```python
from build123d import *

# Parameters (mm, degrees)
F1_DEPTH  = 28.5
F2_R      = 0.5
F3_R      = 3
F4_DEPTH  = 7.9
F5_R      = 2.499
F5_R_2    = 1.999
F6_DEPTH  = 14.8
F7_R      = 2.75
F7_R_2    = 2.499
F7_R_3    = 1.999
F8_DEPTH  = 1
F10_DEPTH = 3.5
F11_R     = 0.15
F12_R     = 0.15


# Not quite as in the source:
# - a feature names something its author has since deleted; it is built from what else it names


with BuildPart() as f1:
    # F0 (on Front) → F1 (new body, symmetric)
    with BuildSketch(Plane.XZ):
        with BuildLine():
            Line((-0.9, 0.9), (-2.3313088598, 0.9))
            ThreePointArc((-2.3313088598, 0.9), (-2.499, 0), (-2.3313088598, -0.9))
            Line((-2.3313088598, -0.9), (-0.9, -0.9))
            Line((-0.9, -0.9), (-0.9, -2.3313088598))
            ThreePointArc((-0.9, -2.3313088598), (0, -2.499), (0.9, -2.3313088598))
            Line((0.9, -2.3313088598), (0.9, -0.9))
            Line((0.9, -0.9), (2.3313088598, -0.9))
            ThreePointArc((2.3313088598, -0.9), (2.499, 0), (2.3313088598, 0.9))
            Line((2.3313088598, 0.9), (0.9, 0.9))
            Line((0.9, 0.9), (0.9, 2.3313088598))
            ThreePointArc((0.9, 2.3313088598), (0, 2.499), (-0.9, 2.3313088598))
            Line((-0.9, 2.3313088598), (-0.9, 0.9))
        make_face()
    extrude(amount=F1_DEPTH, both=True)

    # F2
    f2_edges = [f1.edges().sort_by_distance(p)[0] for p in [
        (0.9, -28.5, 1.615654),
        (-0.9, -28.5, 1.615654),
        (1.615654, -28.5, 0.9),
        (1.615654, -28.5, -0.9),
        (0.9, -28.5, -1.615654),
        (-0.9, -28.5, -1.615654),
        (-1.615654, -28.5, -0.9),
        (-1.615654, -28.5, 0.9),
    ]]
    fillet(f2_edges, radius=F2_R)

    # F3 (on face) → F4 (join)
    with BuildSketch(Plane(origin=(0, 28.5, 0), x_dir=(-1, 0, 0), z_dir=(0, 1, 0))):
        Circle(F3_R)
        with BuildLine():
            Line((-2.3313088598, 0.9), (-0.9, 0.9))
            Line((-0.9, 0.9), (-0.9, 2.3313088598))
            ThreePointArc((-0.9, 2.3313088598), (0, 2.499), (0.9, 2.3313088598))
            Line((0.9, 2.3313088598), (0.9, 0.9))
            Line((0.9, 0.9), (2.3313088598, 0.9))
            ThreePointArc((2.3313088598, 0.9), (2.499, 0), (2.3313088598, -0.9))
            Line((2.3313088598, -0.9), (0.9, -0.9))
            Line((0.9, -0.9), (0.9, -2.3313088598))
            ThreePointArc((0.9, -2.3313088598), (0, -2.499), (-0.9, -2.3313088598))
            Line((-0.9, -2.3313088598), (-0.9, -0.9))
            Line((-0.9, -0.9), (-2.3313088598, -0.9))
            ThreePointArc((-2.3313088598, -0.9), (-2.499, 0), (-2.3313088598, 0.9))
        make_face(mode=Mode.SUBTRACT)
        with BuildLine():
            Line((-0.9, 2.3313088598), (-0.9, 0.9))
            Line((-0.9, 0.9), (-2.3313088598, 0.9))
            ThreePointArc((-2.3313088598, 0.9), (-2.499, 0), (-2.3313088598, -0.9))
            Line((-2.3313088598, -0.9), (-0.9, -0.9))
            Line((-0.9, -0.9), (-0.9, -2.3313088598))
            ThreePointArc((-0.9, -2.3313088598), (0, -2.499), (0.9, -2.3313088598))
            Line((0.9, -2.3313088598), (0.9, -0.9))
            Line((0.9, -0.9), (2.3313088598, -0.9))
            ThreePointArc((2.3313088598, -0.9), (2.499, 0), (2.3313088598, 0.9))
            Line((2.3313088598, 0.9), (0.9, 0.9))
            Line((0.9, 0.9), (0.9, 2.3313088598))
            ThreePointArc((0.9, 2.3313088598), (0, 2.499), (-0.9, 2.3313088598))
        make_face()
    extrude(amount=F4_DEPTH)

    # F5 (on face) → F6 (join)
    with BuildSketch(Plane(origin=(0, 36.4, 0), x_dir=(-1, 0, 0), z_dir=(0, 1, 0))):
        Circle(F5_R)
        Circle(F5_R_2, mode=Mode.SUBTRACT)
    extrude(amount=F6_DEPTH)

    # F7 (on face) → F8 (join)
    with BuildSketch(Plane(origin=(0, 51.2, 0), x_dir=(-1, 0, 0), z_dir=(0, 1, 0))):
        Circle(F7_R)
        Circle(F7_R_2, mode=Mode.SUBTRACT)
        Circle(F7_R_2)
        Circle(F7_R_3, mode=Mode.SUBTRACT)
    extrude(amount=F8_DEPTH)

    # F9 (on face) → F10 (cut)
    with BuildSketch(Plane(origin=(0, 52.2, 0), x_dir=(-1, 0, 0), z_dir=(0, 1, 0))):
        with BuildLine():
            ThreePointArc((-1.983305574, -0.25), (-1.999, 0), (-1.983305574, 0.25))
            Line((-1.983305574, 0.25), (-2.7386127875, 0.25))
            ThreePointArc((-2.7386127875, 0.25), (-2.75, 0), (-2.7386127875, -0.25))
            Line((-2.7386127875, -0.25), (-1.983305574, -0.25))
        make_face()
        with BuildLine():
            ThreePointArc((2.7386127875, -0.25), (2.75, 0), (2.7386127875, 0.25))
            Line((2.7386127875, 0.25), (1.983305574, 0.25))
            ThreePointArc((1.983305574, 0.25), (1.999, 0), (1.983305574, -0.25))
            Line((1.983305574, -0.25), (2.7386127875, -0.25))
        make_face()
    extrude(amount=-F10_DEPTH, mode=Mode.SUBTRACT)

    # F11
    f11_edges = [f1.edges().sort_by_distance(p)[0] for p in [
        (2.234885, 48.7, -0.25),
        (2.234885, 48.7, 0.25),
        (-2.234885, 48.7, -0.25),
        (-2.234885, 48.7, 0.25),
    ]]
    fillet(f11_edges, radius=F11_R)

    # F12
    f12_edges = [f1.edges().sort_by_distance(p)[0] for p in [
        (0, 52.2, 2.75),
        (0, 52.2, -2.75),
        (0, 51.2, -2.75),
        (0, 51.2, 2.75),
    ]]
    fillet(f12_edges, radius=F12_R)


solid = f1.part
```
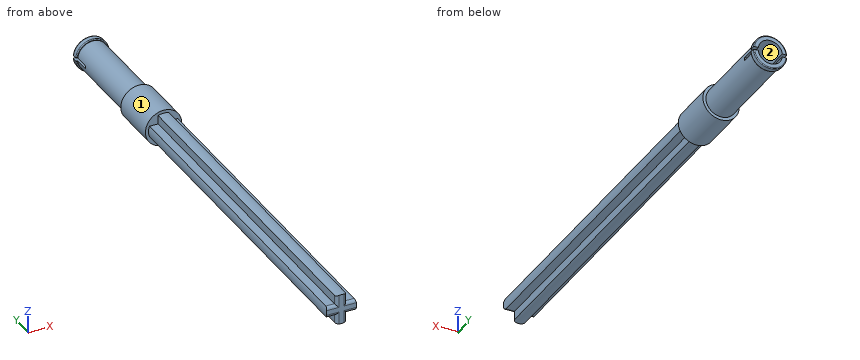
CAD build for the part. Positions are in the model's coordinates, mm. Face numbers are marked on the shaded views. Coordinates: 2 decimals unless noted, no trailing zeros. Order: outer loops, then holes, each group sorted by start corner. A loop starts at its lowest first (then second) coordinate and runs counter-clockwise, first axis right, second up. Notation, with made-up numbers: (-13.75, -20) - (-1.75, -20) arc R21 cw to (-1.75, -7) - close; hole circle Ø4 at (79.25, 32.5). An arc over 180 degrees is marked (long way). Use a Markdown table: item, result. Add a question column.
(1) Saw through at A-A (y = -7). Give the cut face in (x, z), then the cut area to 3 significant figures.
(2) Pull direction X, two halves, no side cores. Call the marked faces 1 and 2: +X half, -X half, draft (parallel to the pull), parting line (faces both ways), or undercut.
(3) Drill centre lines: line 1 along Y through (x, z) = (-2.35, 1); line 2 along Z through (x, y) = (0, 46.5); line 3 along Y through (x, z) = (-1.4, 0.2). Where is each one in solid material? Low to high. Write a range as [from, to].
(4) Flat gauge pins, fed straight in: pin 1 (0.7 mm diameter, centred on x = 1.5, y = -13.5, fed in from -Z); pin 2 (3 mm diameter, centred on y = 13.5, z = -2, fed in from +X); pin 3 (2.5 mm diameter, centred on x = 0, z = 0, fed in from +Y); pin 4 (3 mm diameter, centred on x = 0.5, z = 1.5, fed in from +Y). Where does each tip first touch, or does it go through?
(5) Saw through at B-B (y = 37.5). Give the cut face in (x, z), then the cut area to 3 significant figures.
Solved:
| question | item | result |
|---|---|---|
| 1 | outline | (-2.33, -0.9) - (-0.9, -0.9) - (-0.9, -2.33) arc R2.5 ccw to (0.9, -2.33) - (0.9, -0.9) - (2.33, -0.9) arc R2.5 ccw to (2.33, 0.9) - (0.9, 0.9) - (0.9, 2.33) arc R2.5 ccw to (-0.9, 2.33) - (-0.9, 0.9) - (-2.33, 0.9) arc R2.5 ccw to start |
| 1 | area | 14.4 mm² |
| 2 | face 1 | parting line |
| 2 | face 2 | undercut |
| 3 | line 1 | y = [28.5, 36.4], [51.2, 52.2] |
| 3 | line 2 | z = [-2.5, -2], [2, 2.5] |
| 3 | line 3 | y = [-28.5, 36.4] |
| 4 | pin 1 | stops at z = -0.9 |
| 4 | pin 2 | stops at x = 2.45 |
| 4 | pin 3 | stops at y = 36.4 |
| 4 | pin 4 | stops at y = 52.2 |
| 5 | outline | circle Ø5 at (0, 0); hole circle Ø4 at (0, 0) |
| 5 | area | 7.07 mm² |
